```python
from build123d import *

# Parameters (mm, degrees)
F0_W     = 838.2
F0_H     = 2438.4
F1_DEPTH = 152.4
F2_W     = 752.025268
F2_H     = 339.915395
F3_DEPTH = 50.8
F4_W     = 174.812899
F4_H     = 339.915395
F5_DEPTH = 254


with BuildPart() as f1:
    # F0 (on Front) → F1 (new body)
    with BuildSketch(Plane.XZ):
        Rectangle(F0_W, F0_H)
    extrude(amount=F1_DEPTH)

    # F2 (on face) → F3 (join)
    with BuildSketch(Plane.XZ.offset(152.4)):
        with Locations((-217.900265, -634.607195)):
            Rectangle(F2_W, F2_H)
    extrude(amount=F3_DEPTH)

    # F4 (on face) → F5 (join)
    with BuildSketch(Plane(origin=(0, -152.4, 0), x_dir=(-1, 0, 0), z_dir=(0, 1, 0))):
        with Locations((506.506449, -634.607195)):
            Rectangle(F4_W, F4_H)
    extrude(amount=F5_DEPTH)


solid = f1.part
```
Build history of the part. All positions in model axes, mm. A direction names the side the tool comes from. Round coordinates to 2 decimals unless told otherwise and drop trailing zeros. Loops run counter-clockwise (first coordinate to the right, second up) from the corner with the lowest first, then second, coordinate; pieces in that order, holes last.
Item 1: Pin check, flat tips, straight feed: P1, Ø2, axis at x = -258, y = -165, coming from the -Z side; P2, Ø1.5, axis at x = -205.5, z = 181.5, coming from the +Y side; P3, Ø10, axis at y = -92, z = -356.5, coming from the -X side. Stop position of each tip, or through.
Item 2: Saw through at B-B (x = -369.5). List the corners of the cut face in (y, z).
Item 3: Saw through at A-A (z = -751.5). List the corners of the cut face in (x, y).
Item 4: Saw through at D-D (z = -437.5). List the corners of the cut face in (x, y), then the cut area to 3 significant figures.
Item 5: Which spindle directions (+Z, -Z, +X, -X, +Y, -Y) get a long thin tool onto all of the face, cutting with end or side? Do faces 1 (the face through (158.112, -177, -637)), 2 (the face through (-419.1, -75, 365)), 3 (the face through (-419.1, 50, -637)), 4 (the face through (-419.1, -75, -1015)). Say none if no direction does.
Item 6: Saw through at C-C (y = 41). List the corners of the cut face in (x, z).
Item 7: Drill centre lines: line 1 along X through (y, z) = (-104, -463.5); line 2 along Y through (x, z) = (149.5, -788.5); line 3 along Z through (x, y) = (-471.5, 81.5). Where is each one in solid material? Low to high.
Worked answers:
1. P1: stops at z = -804.56
1. P2: stops at y = 0
1. P3: stops at x = -419.1
2. outline: (-203.2, -804.56) - (-152.4, -804.56) - (-152.4, -1219.2) - (0, -1219.2) - (0, 1219.2) - (-152.4, 1219.2) - (-152.4, -464.65) - (-203.2, -464.65) - close
3. outline: (-593.91, -203.2) - (158.11, -203.2) - (158.11, -152.4) - (419.1, -152.4) - (419.1, 0) - (-419.1, 0) - (-419.1, 101.6) - (-593.91, 101.6) - close
4. outline: (-419.1, -152.4) - (419.1, -152.4) - (419.1, 0) - (-419.1, 0) - close
4. area: 128,000 mm2
5. face 1: +Z, -Z, +X, -Y
5. face 2: +Z, -X, +Y, -Y
5. face 3: +Z, -Z, +X, +Y
5. face 4: -Z, -X, +Y, -Y
6. outline: (-593.91, -804.56) - (-419.1, -804.56) - (-419.1, -464.65) - (-593.91, -464.65) - close
7. line 1: x = -419.1 to 419.1
7. line 2: y = -203.2 to 0
7. line 3: z = -804.56 to -464.65
